Verification items for the finished model (mm, model axes). Face numbers are marked on the shaded views. Give positions to 0.01 mm unless a question says otherwise; leave off trailing zeros. Order: outer loops, then holes, each group sorted by start corner. A loop starts at its lowest first (then second) coordinate and runs counter-clockwise, first axis right, second up.
(1) Sectioned sample at C-C on y = 11.75. Record the cut outline in (x, z), plus the area to 3 significant figures.
(2) Scan lines: L1, parallel to Y at x = -4.5, z = -28; L2, parallel to X at y = 2.5, z = -30; L3, parallel to X at y = 13.5, z = 0. Record each from-to range of solid material in increasing order.
(3) Sectioned sample at A-A on x = 0. Record the cut outline in (y, z).
(4) Sectioned sample at D-D on x = -4. Record the cut outline in (y, z).
(5) Sectioned sample at B-B on z = -20. Record the cut outline in (x, y).
(6) Mould release check, pull along Y, two halves, no side actions. Record for the marked faces 1, 2, 3 and 4: pulls with the +Y half, pulls with the -Y half, needs draft (parallel to the pull), parting line crosses it, or undercut.
```python
from build123d import *

# Parameters (mm, degrees)
ESQUISSE1_R        = 1.95
ESQUISSE1_R_2      = 2.05
BOSS_EXTRU_1_DEPTH = 5
ESQUISSE2_R        = 2.05
BOSS_EXTRU_2_DEPTH = 8
BOSS_EXTRU_3_START = 8
ESQUISSE3_R        = 1.95
ESQUISSE3_R_2      = 2.05
BOSS_EXTRU_3_DEPTH = 5


with BuildPart() as part:
    # Esquisse1 → Boss.-Extru.1 (new body)
    with BuildSketch(Plane(origin=(0, 0, 0), x_dir=(1, 0, 0), z_dir=(0, 1, 0))):
        with BuildLine():
            Line((-5, 0), (-5, 30))
            ThreePointArc((-5, 30), (0, 35), (5, 30))
            Line((5, 30), (5, 0))
            ThreePointArc((5, 0), (0, -5), (-5, 0))
        make_face()
        with Locations(Location((0, 30, 0), (0, 0, 270))):
            Circle(ESQUISSE1_R, mode=Mode.SUBTRACT)
        with Locations(Location((0, 0, 0), (0, 0, 270))):
            Circle(ESQUISSE1_R_2, mode=Mode.SUBTRACT)
    extrude(amount=BOSS_EXTRU_1_DEPTH)

    # Esquisse2 → Boss.-Extru.2 (add)
    with BuildSketch(Plane(origin=(0, 5, 0), x_dir=(1, 0, 0), z_dir=(0, 1, 0))):
        with BuildLine():
            Line((-5, 0), (-5, 6))
            ThreePointArc((-5, 6), (0, 11), (5, 6))
            Line((5, 6), (5, 0))
            ThreePointArc((5, 0), (0, -5), (-5, 0))
        make_face()
        with Locations(Location((0, 0, 0), (0, 0, 270))):
            Circle(ESQUISSE2_R, mode=Mode.SUBTRACT)
    extrude(amount=BOSS_EXTRU_2_DEPTH)

    # Esquisse3 → Boss.-Extru.3 (add)
    # profile 1 of 2: a face of its own
    with BuildSketch(Plane(origin=(0, 5, 0), x_dir=(1, 0, 0), z_dir=(0, 1, 0)).offset(BOSS_EXTRU_3_START)):
        with BuildLine():
            Line((-5, 30), (-5, 6))
            ThreePointArc((-5, 6), (0, 11), (5, 6))
            Line((5, 6), (5, 30))
            ThreePointArc((5, 30), (0, 35), (-5, 30))
        make_face()
        with Locations(Location((0, 30, 0), (0, 0, 270))):
            Circle(ESQUISSE3_R, mode=Mode.SUBTRACT)
    # profile 2 of 2: a face of its own
    with BuildSketch(Plane(origin=(0, 5, 0), x_dir=(1, 0, 0), z_dir=(0, 1, 0)).offset(BOSS_EXTRU_3_START)):
        with BuildLine():
            Line((-5, 6), (-5, 0))
            ThreePointArc((-5, 0), (0, -5), (5, 0))
            Line((5, 0), (5, 6))
            ThreePointArc((5, 6), (0, 11), (-5, 6))
        make_face()
        with Locations(Location((0, 0, 0), (0, 0, 270))):
            Circle(ESQUISSE3_R_2, mode=Mode.SUBTRACT)
    extrude(amount=BOSS_EXTRU_3_DEPTH)


solid = part.part
```
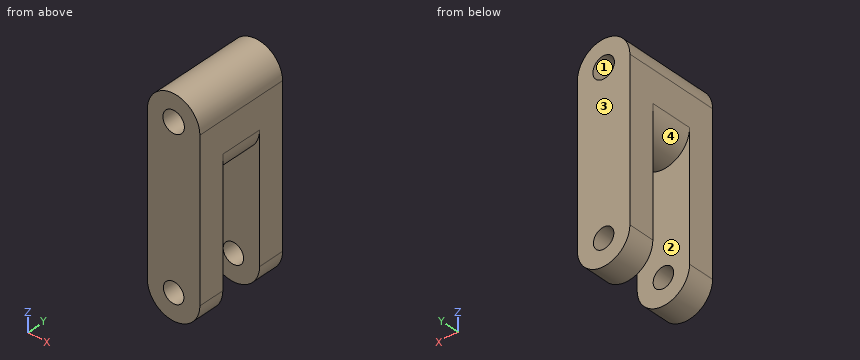
Ans:
1. outline: (-5, -6) arc R5 ccw to (5, -6) - (5, 0) arc R5 ccw to (-5, 0) - close; hole circle Ø4.1 at (0, 0)
1. area: 125 mm2
2. L1: y = 0 to 5, 13 to 18
2. L2: x = -5 to -1.95, 1.95 to 5
2. L3: x = -5 to -2.05, 2.05 to 5
3. outline: (0, -35) - (5, -35) - (5, -31.95) - (0, -31.95) - close; (0, -28.05) - (5, -28.05) - (5, -11) - (13, -11) - (13, -28.05) - (18, -28.05) - (18, -2.05) - (0, -2.05) - close; (0, 2.05) - (18, 2.05) - (18, 5) - (0, 5) - close; (13, -35) - (18, -35) - (18, -31.95) - (13, -31.95) - close
4. outline: (0, -33) - (5, -33) - (5, -9) - (13, -9) - (13, -33) - (18, -33) - (18, 3) - (0, 3) - close
5. outline: (-5, 0) - (5, 0) - (5, 5) - (-5, 5) - close; (-5, 13) - (5, 13) - (5, 18) - (-5, 18) - close
6. face 1: needs draft
6. face 2: undercut
6. face 3: pulls with the +Y half
6. face 4: undercut
